Here's how the part is built. I have some questions about the finished solid (model axes, mm). Round coordinates to 2 decimals unless told otherwise and drop trailing zeros. Loops run counter-clockwise (first coordinate to the right, second up) from the corner with the lowest first, then second, coordinate; pieces in that order, holes last. Notation, with made-up numbers: (74, 70.25) - (112, 70.25) arc R15 cw to (112, 74.25) - close; hole circle Ø2 at (2, 89.5). An arc over 180 degrees is marked (long way). Return JSON: item names as keys, results as strings. Group by question number.
```python
from build123d import *

# Parameters (mm, degrees)
F0_R     = 20
F1_DEPTH = 25
F4_COUNT = 3


with BuildPart() as f1:
    # F0 (on Front) → F1 (new body, symmetric)
    with BuildSketch(Plane.XZ):
        Circle(F0_R)
    extrude(amount=F1_DEPTH, both=True)


with BuildPart() as f4_1:
    # F4: instance of F1
    add(f1.part.rotate(Axis((-10, 10, 10), (-0.5773502692, 0.5773502692, 0.5773502692)), 1 * 360 / F4_COUNT))


with BuildPart() as f4_2:
    # F4: instance of F1
    add(f1.part.rotate(Axis((-10, 10, 10), (-0.5773502692, 0.5773502692, 0.5773502692)), 2 * 360 / F4_COUNT))

    # F5: intersect F4_1, F1
    add(f4_1.part, mode=Mode.INTERSECT)
    add(f1.part, mode=Mode.INTERSECT)


solid = f4_2.part
```
Q1. Imagine slicing it at D-D, the plane y = 15. List the corners of the cut face in (x, z) for me.
Q2. Imagine slicing it at B-B, the plane y = -4. List the corners of the cut face in (x, z) for me, and give its area (3 significant figures).
Q3. Imagine slicing it at C-C, the plane x = -16.5. List the corners of the cut face in (y, z) for me.
Q4. Will these pins go through, and if not, where does the flat tip stop? pin 1 Ø1.5 at (x, z) = (-7, -7.5) entering from -Y; pin 2 Ø12 at (x, z) = (-1, -8) entering from +Y; pin 3 Ø10 at (x, z) = (-2, -12) entering from +Y (3 decimals).
Q5. Please list where these lines run through material, in increasing order: line 1 (Z direction, x = -9.5, y = 5); line 2 (Z direction, x = 13, y = 3.5); line 3 (X direction, y = -1, z = 14.5).
Q6. Imagine slicing it at A-A, the plane x = 2. List the corners of the cut face in (y, z) for me, and give its area (3 significant figures).
Output values:
{
 "1": {"outline": "(-13.23, -13.23) - (13.23, -13.23) - (13.23, 13.23) - (-13.23, 13.23) - close"},
 "2": {"outline": "(-19.6, -4) arc R20 ccw to (-4, -19.6) - (4, -19.6) arc R20 ccw to (19.6, -4) - (19.6, 4) arc R20 ccw to (4, 19.6) - (-4, 19.6) arc R20 ccw to (-19.6, 4) - close", "area": "1,250 mm^2"},
 "3": {"outline": "(-11.3, -11.3) - (11.3, -11.3) - (11.3, 11.3) - (-11.3, 11.3) - close"},
 "4": {"pin 1": "stops at y = -18.81", "pin 2": "stops at y = 19.9", "pin 3": "stops at y = 18.735"},
 "5": {"line 1": "z = -17.6 to 17.6", "line 2": "z = -15.2 to 15.2", "line 3": "x = -13.77 to 13.77"},
 "6": {"outline": "(-19.9, -2) arc R20 ccw to (-2, -19.9) - (2, -19.9) arc R20 ccw to (19.9, -2) - (19.9, 2) arc R20 ccw to (2, 19.9) - (-2, 19.9) arc R20 ccw to (-19.9, 2) - close", "area": "1,260 mm^2"}
}
